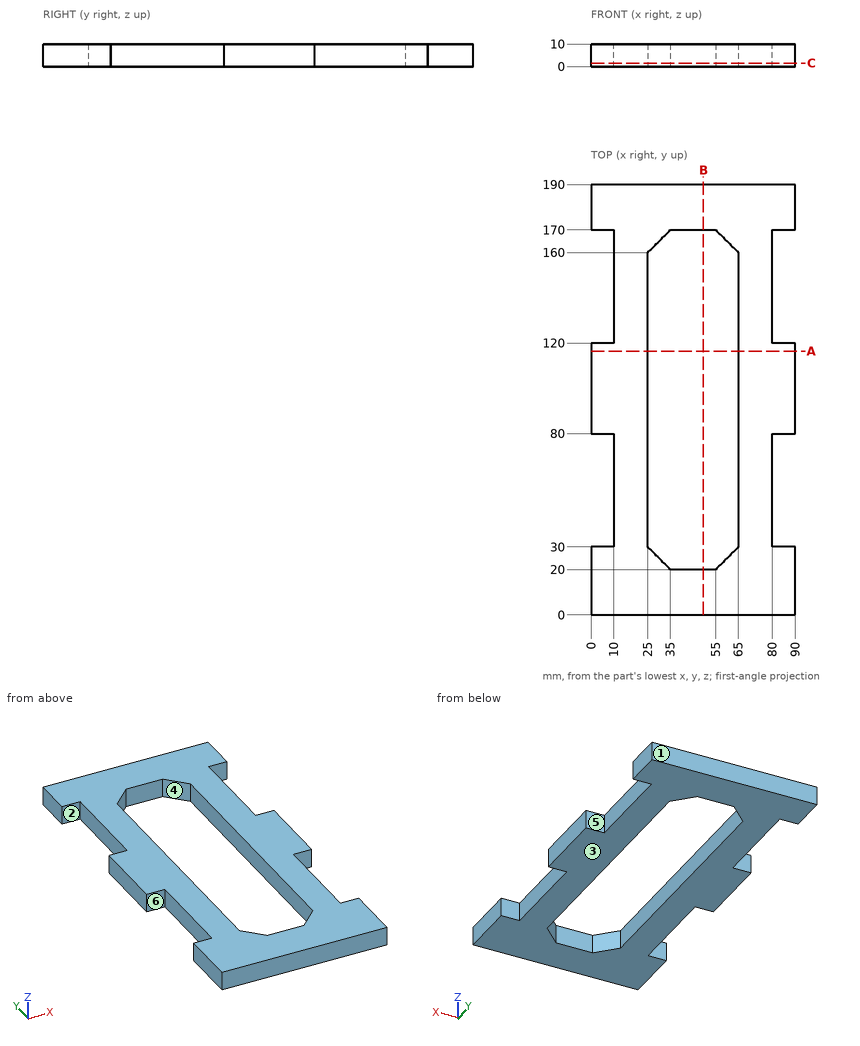
Geometry: see drawing. Coordinates: mm, zero at the bounding-box minimum. A direction names the side the tool comes from. Give positions to 0.01 mm unless a question says otherwise; leave off trailing zeros. Order: outer loops, then holes, each group sorted by start corner. A loop starts at its lowest first (then second) coordinate and runs counter-clockwise, first axis right, second up.
Q1. Draft query along Y for the marked faces 1, 2 and 3. Return one class per face: +Y half, -Y half, draft (parallel to the pull), parting line (faces both ways), or undercut.
Checked values:
face 1: +Y half
face 2: undercut
face 3: draft
Q2. Section C-C on z = 1.5. Output: boundary loops of the cut face in (x, y), and give its area (3 significant figures).
Checked values:
outline: (0, 0) - (90, 0) - (90, 30) - (80, 30) - (80, 80) - (90, 80) - (90, 120) - (80, 120) - (80, 170) - (90, 170) - (90, 190) - (0, 190) - (0, 170) - (10, 170) - (10, 120) - (0, 120) - (0, 80) - (10, 80) - (10, 30) - (0, 30) - close; hole (25, 30) - (35, 20) - (55, 20) - (65, 30) - (65, 160) - (55, 170) - (35, 170) - (25, 160) - close
area: 9,300 mm2
Q3. Contact query for flat-ended pins moving along their axis: pin 1 Ø1 at (y, z) = (69, 2) entering from +X; pin 2 Ø3 at (y, z) = (120, 7) entering from -X; pin 3 Ø5 at (y, z) = (135.5, 3.5) entering from -X. Output: stop coordinate, or through.
Checked values:
pin 1: stops at x = 80
pin 2: stops at x = 0
pin 3: stops at x = 10
Q4. Section A-A on y = 116.5. Output: boundary loops of the cut face in (x, z).
Checked values:
outline: (0, 0) - (25, 0) - (25, 10) - (0, 10) - close; (65, 0) - (90, 0) - (90, 10) - (65, 10) - close
Q5. Ray query, probe 1 along Y at (x, z) = (6.5, 3.5); probe 2 along X at (y, z) = (79, 3); probe 3 along X at (y, z) = (104, 2.5). Return the intervals inside material, ascending.
Checked values:
probe 1: y = 0 to 30, 80 to 120, 170 to 190
probe 2: x = 10 to 25, 65 to 80
probe 3: x = 0 to 25, 65 to 90
Q6. Section B-B on x = 49.5. Output: boundary loops of the cut face in (y, z), and give its area (3 significant figures).
Checked values:
outline: (0, 0) - (20, 0) - (20, 10) - (0, 10) - close; (170, 0) - (190, 0) - (190, 10) - (170, 10) - close
area: 400 mm2
Q7. Set-up query: the marked faces 4, 5 and 6. Return all of +Z, -Z, +X, -X, +Y, -Y with unobstructed straight access to the full face (end or side cutting, diameter ignored); none if empty.
Checked values:
face 4: +Z, -Z
face 5: +Z, -Z, +X
face 6: +Z, -Z, -X
